The listing builds one solid part. Answer for the finished solid, in the listing's coordinates (mm). Give positions to 0.01 mm unless a question says otherwise; leave off trailing zeros. Order: outer loops, then holes, each group sorted by start corner. A loop starts at its lowest first (then second) coordinate and runs counter-clockwise, first axis right, second up. Notation, with made-up numbers: (60.5, 23.25) - (85.5, 23.25) arc R27 ccw to (85.5, 53.25) - close; hole circle Ø5 at (-15.75, 10.5). An arc over 180 degrees is marked (long way). Answer as a JSON object with one key per item and string values. Group by question number.
Q1. Consider line 1 (Z direction, x = -2, y = 5); line 2 (Z direction, x = -8, y = -4); line 3 (Y direction, x = 0.75, z = -48.5). Determine where each line is inside the solid, lowest interval first.
Q2. A cutting plane is placed at A-A, the plane z = -2.5. Give the vertices of the cut face in (x, y) (3 decimals), and give its area (3 significant figures).
Q3. Given pin 1 (10 mm diameter, centred on y = -3, z = -87.5, fed in from -X) (3 decimals); pin 2 (4 mm diameter, centred on y = 7.5, z = 48, fed in from -X) (1 decimal), each flat-ended and moving along its own axis, determine where each tip first touches the part or whether it passes through.
from build123d import *

# Parameters (mm, degrees)
SKETCH1_R           = 0.925
BOSS_EXTRUDE1_DEPTH = 35.25
SKETCH2_R           = 2
BOSS_EXTRUDE2_DEPTH = 1
CHAMFER1_SIZE       = 0.5
FILLET1_R           = 0.1
SCALE1_SCALE        = 5


with BuildPart() as part:
    # Sketch1 → Boss-Extrude1 (new body)
    with BuildSketch(Plane.XY):
        Circle(SKETCH1_R)
    extrude(amount=BOSS_EXTRUDE1_DEPTH)

    # Sketch2 → Boss-Extrude2 (add)
    with BuildSketch(Plane.XY.offset(35.25)):
        Circle(SKETCH2_R)
    extrude(amount=BOSS_EXTRUDE2_DEPTH)

    # Chamfer1
    chamfer1_edges = [part.edges().sort_by_distance(p)[0] for p in [
        (-2, 0, 36.25),
    ]]
    chamfer(chamfer1_edges, length=CHAMFER1_SIZE)

    # Mirror1: part across plane


with BuildPart() as part_1:
    add(part.part)
    add(part.part.mirror(Plane.XY))

    # Fillet1
    fillet1_edges = [part_1.edges().sort_by_distance(p)[0] for p in [
        (-1.5, 0, 36.25),
        (-2, 0, 35.75),
        (-0.925, 0, 35.25),
        (-2, 0, 35.25),
    ]]
    fillet(fillet1_edges, radius=FILLET1_R)


with BuildPart() as part_2:
    # Scale1: scaled about (-2.8e-08, 0, -0.003118898)
    add(part_1.part.scale(SCALE1_SCALE).moved(Location((1.12e-07, 0, 0.012475592))))


solid = part_2.part
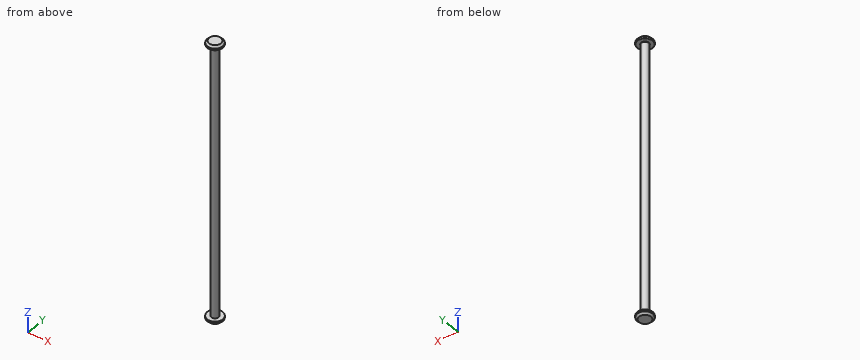
Reply:
{
 "1": {"line 1": "z = -181.24 to -176.24, 176.26 to 181.26", "line 2": "z = -179.79 to -176.24, 176.26 to 179.82", "line 3": "y = -4.56 to 4.56"},
 "2": {"outline": "circle Ø9.25 at (0, 0)", "area": "67.2 mm^2"},
 "3": {"pin 1": "stops at x = -4.625", "pin 2": "passes through"}
}
